Part model, mm, in its own coordinate system. A direction names the side the tool comes from. Give positions to 0.01 mm unless a question says otherwise; leave off trailing zeros. Order: outer loops, then holes, each group sorted by start corner. A loop starts at its lowest first (then second) coordinate and runs counter-clockwise, first axis right, second up. Notation, with made-up numbers: (-0.75, 72) - (54.25, 72) arc R20 ccw to (54.25, 94) - close; hole circle Ø6 at (-24.5, -20.5). An arc over 180 degrees is marked (long way). Use one line per item in the form item = value. Start each with the question number.
1. Band-saw the part on A-A, the plane x = -95. List the corners of the cut face in (y, z), plus the area to 3 significant figures.
2. Band-saw the part on C-C, the plane y = -38. List the corners of the cut face in (x, z), plus the area to 3 significant figures.
3. Pin check, flat tip, straight feed: P1, Ø1, axis at x = -33, y = -40, coming from the -Z side. Stop position of the tip, or through.
4. Pull direction X, two halves, no side cores. Call faces 4 (the face through (-76.426, -20.265, 70.492)), 5 (the face through (-61, 24, 80)), 6 (the face through (0, -1, 39)): +X half, -X half, draft (parallel to the pull), parting line (faces both ways), or undercut.
5. Drill centre lines: line 1 (X direction, y = -6, z = 77); line 2 (Y direction, x = -40, z = 18.5); line 3 (Z direction, x = -35.5, y = 24). Where is each one in solid material? Low to high.
6. Tool access for faces 1 (the face through (-48.027, -35.392, 53.572)), 2 (the face through (-103.496, -20.21, 70.547)), 3 (the face through (-76.5, -53.55, 37.21)): list every direction of +Z, -Z, +X, -X, +Y, -Y with a clear straight run to the whole face (end or side of a thin tool).
7. Band-saw the part on B-B, the plane z = 9. List the corners of the cut face in (x, y).
8. Band-saw the part on D-D, the plane x = -40. List the corners of the cut face in (y, z), plus the area to 3 significant figures.
from build123d import *

# Parameters (mm, degrees)
F0_W     = 120
F0_H     = 80
F1_DEPTH = 62.5
F2_SIZE  = 50
F3_T     = -2.5
F5_DEPTH = 25


with BuildPart() as f1:
    # F0 (on Front) → F1 (new body, symmetric)
    with BuildSketch(Plane.XZ):
        with Locations((-60, 40)):
            Rectangle(F0_W, F0_H)
    extrude(amount=F1_DEPTH, both=True)

    # F2
    f2_edges = [f1.edges().sort_by_distance(p)[0] for p in [
        (-60, -62.5, 80),
    ]]
    chamfer(f2_edges, length=F2_SIZE)

    # F3
    f3_openings = [f1.faces().sort_by_distance(p)[0] for p in [
        (-60, 0, 0),
    ]]
    offset(amount=F3_T, openings=f3_openings)

    # F4 (on face) → F5 (cut)
    with BuildSketch(Plane(origin=(0, -46.25, 46.25), x_dir=(1, 0, 0), z_dir=(0, -0.707107, 0.707107))):
        with BuildLine():
            Line((-80, 37.01903), (-100, 37.01903))
            ThreePointArc((-100, 37.01903), (-103.535534, 35.554564), (-105, 32.01903))
            Line((-105, 32.01903), (-105, -7.98097))
            ThreePointArc((-105, -7.98097), (-103.535534, -11.516504), (-100, -12.98097))
            Line((-100, -12.98097), (-80, -12.98097))
            ThreePointArc((-80, -12.98097), (-76.464466, -11.516504), (-75, -7.98097))
            Line((-75, -7.98097), (-75, 32.01903))
            ThreePointArc((-75, 32.01903), (-76.464466, 35.554564), (-80, 37.01903))
        make_face()
    extrude(amount=-F5_DEPTH, mode=Mode.SUBTRACT)


solid = f1.part
From the geometry:
q1.outline = (-62.5, 0) - (-60, 0) - (-60, 28.96) - (-53.66, 35.3) - (-55.43, 37.07) - (-62.5, 30) - close; (-20.07, 72.43) - (-18.31, 70.66) - (-11.46, 77.5) - (60, 77.5) - (60, 0) - (62.5, 0) - (62.5, 80) - (-12.5, 80) - close
q1.area = 503 mm²
q2.outline = (-120, 0) - (-117.5, 0) - (-117.5, 50.96) - (-105, 50.96) - (-105, 54.5) - (-120, 54.5) - close; (-75, 50.96) - (-2.5, 50.96) - (-2.5, 0) - (0, 0) - (0, 54.5) - (-75, 54.5) - close
q2.area = 573 mm²
q3.P1 = 48.46
q4.face_4 = undercut
q4.face_5 = draft
q4.face_6 = +X half
q5.line_1 = -120 to -117.5, -2.5 to 0
q5.line_2 = -62.5 to -60, 60 to 62.5
q5.line_3 = 77.5 to 80
q6.face_1 = -Z
q6.face_2 = -Z, -Y
q6.face_3 = +Z
q7.outline = (-120, -62.5) - (0, -62.5) - (0, 62.5) - (-120, 62.5) - close; hole (-117.5, -60) - (-2.5, -60) - (-2.5, 60) - (-117.5, 60) - close
q8.outline = (-62.5, 0) - (-60, 0) - (-60, 28.96) - (-11.46, 77.5) - (60, 77.5) - (60, 0) - (62.5, 0) - (62.5, 80) - (-12.5, 80) - (-62.5, 30) - close
q8.area = 628 mm²
